```python
from build123d import *

# Parameters (mm, degrees)
F0_W     = 1050
F0_H     = 500
F1_DEPTH = 750
F2_W     = 625.638008
F2_H     = 585.840762
F3_DEPTH = 500
F4_W     = 356.15398
F4_H     = 580.154359
F5_DEPTH = 54.955602


with BuildPart() as f1:
    # F0 (on Top) → F1 (new body)
    with BuildSketch(Plane.XY):
        with Locations((-525, 250)):
            Rectangle(F0_W, F0_H)
    extrude(amount=F1_DEPTH)

    # F2 (on face) → F3 (cut, through all)
    with BuildSketch(Plane.XZ):
        with Locations((-367.774606, 292.920381)):
            Rectangle(F2_W, F2_H)
    extrude(amount=-F3_DEPTH, mode=Mode.SUBTRACT)

    # F4 (on face) → F5 (cut, through all)
    with BuildSketch(Plane.YZ):
        with Locations((252.290092, 290.077179)):
            Rectangle(F4_W, F4_H)
    extrude(amount=-F5_DEPTH, mode=Mode.SUBTRACT)


solid = f1.part
```
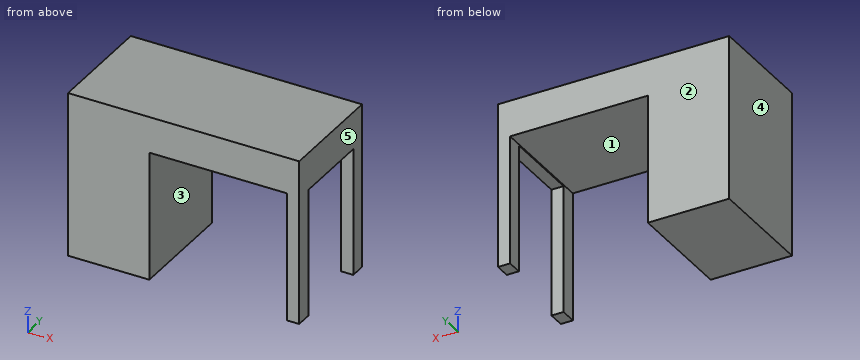
Design review of the part built by this model. Coordinates are the model's own, in mm. Face numbers are marked on the shaded views. A direction names the side the tool comes from. Coordinates: 2 decimals unless noted, no trailing zeros. Write each loop counter-clockwise with the first axis right and the second up, starting at its lowest first coordinate (ties: lowest second). Pieces come first, ordered by that corner, then holes.
1) To check wall thickness, follow L1, parallel to X at y = 43.5, z = 567; L2, parallel to Z at x = -206.5, y = 124.5; L3, parallel to X at y = 291, z = 566.5. State the ranges of each line that lie inside material, in increasing order.
2) Mouldability with a two-part tool opening along X and no side actions: class the marked faces 3, 4 and 5 as +X half, -X half, draft (parallel to the pull), parting line (faces both ways), or undercut.
3) Add section C-C (x = -511.5). Write out the cut boundary in (y, z), plus the area to 3 significant figures.
4) Add section B-B (y = 296.5). Write out the cut boundary in (x, z), plus the area to 3 significant figures.
5) Add section D-D (y = 452). Write out the cut boundary in (x, z), plus the area to 3 significant figures.
6) Add section A-A (z = 363). Write out the cut boundary in (x, y), plus the area to 3 significant figures.
7) Machinability: for the marked faces 1 and 2, which of the approach directions +Z, -Z, +X, -X, +Y, -Y give a long, thin tool a straight path to every point of the face, cutting with its end or side? Answer none if there is none.
8) Insertion check: pin 1 (1 mm diameter, centred on y = 127, z = 497.5, fed in from +X); pin 2 (16.5 mm diameter, centred on x = -28, y = 219, fed in from -Z). Each pin has a flat end and moves straight along its axis. Give the tip position at first contact, or say it passes through.
Check result:
1. L1: x = -1050 to -680.59, -54.96 to 0
1. L2: z = 585.84 to 750
1. L3: x = -1050 to -680.59
2. face 3: undercut
2. face 4: -X half
2. face 5: +X half
3. outline: (0, 585.84) - (500, 585.84) - (500, 750) - (0, 750) - close
3. area: 82,100 mm2
4. outline: (-1050, 0) - (-680.59, 0) - (-680.59, 585.84) - (-54.96, 585.84) - (-54.96, 580.15) - (0, 580.15) - (0, 750) - (-1050, 750) - close
4. area: 389,000 mm2
5. outline: (-1050, 0) - (-680.59, 0) - (-680.59, 585.84) - (-54.96, 585.84) - (-54.96, 0) - (0, 0) - (0, 750) - (-1050, 750) - close
5. area: 421,000 mm2
6. outline: (-1050, 0) - (-680.59, 0) - (-680.59, 500) - (-1050, 500) - close; (-54.96, 0) - (0, 0) - (0, 74.21) - (-54.96, 74.21) - close; (-54.96, 430.37) - (0, 430.37) - (0, 500) - (-54.96, 500) - close
6. area: 193,000 mm2
7. face 1: -Z, +Y, -Y
7. face 2: +Z, -Z, +X, -X, +Y
8. pin 1: stops at x = -680.59
8. pin 2: stops at z = 580.15
